Could you check a few things on this drawing? It's one solid part, dimensions in mm from its lowest x, y, z. A direction names the side the tool comes from. Round coordinates to 2 decimals unless told otherwise and drop trailing zeros. Order: outer loops, then holes, each group sorted by start corner. A loop starts at its lowest first (then second) coordinate and runs counter-clockwise, first axis right, second up.
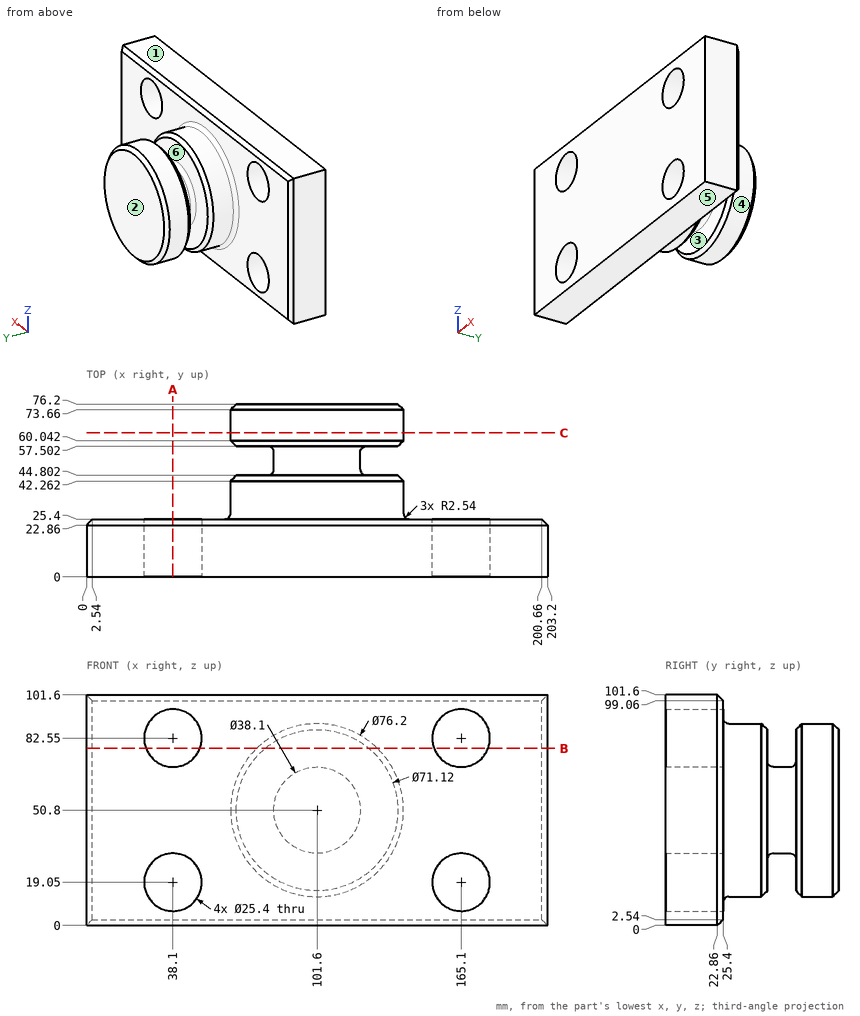
(1) I want a section at B-B, the plane z = 78. Give the number of separate pieces and of enclosed holes in the cut face, plus the area to 3 significant figures.
(2) I want a section at A-A, the plane x = 38.1. List the corners of the cut face in (y, z) for me, plus the area to 3 significant figures.
(3) I'm going to push flat-ended pins straight in: pin 1 Ø4 at (y, z) = (56, 67) entering from +X; pin 2 Ø2 at (x, z) = (132.5, 22.5) entering from -Y; pin 3 Ø1 at (y, z) = (50, 33.5) entering from -X; pin 4 Ø1.5 at (y, z) = (58, 21.5) entering from +X. Where does each tip first touch, or does it pass through?
(4) I want a section at C-C, the plane y = 63.5. List the corners of the cut face in (x, z) for me, plus the area to 3 significant figures.
(5) If we mould it in two halves opening along Y, with no side actions, what happens to the marked faces 1, 2 and 3? For each: pulls with the +Y half, pulls with the -Y half, needs draft (parallel to the pull), parting line crosses it, or undercut.
(6) On a 3-axis mill with a long thin cutter (end or side, diameter ignored), from which of +Z, -Z, +X, -X, +Y, -Y can I reach the whole of each face in a straight line? I mean the marked faces 4, 5 and 6. Say none if no direction works.
(7) Please list where these lines run through material, in increasing order: probe 1 along Z at (x, y) = (38.1, 7.5); probe 2 along X at (y, z) = (11, 82); probe 3 along X at (y, z) = (23.5, 83).
Ans:
1. separate pieces: 4
1. enclosed holes: 0
1. area: 5,960 mm2
2. outline: (0, 0) - (22.86, 0) - (25.4, 2.54) - (25.4, 6.35) - (0, 6.35) - close; (0, 31.75) - (25.4, 31.75) - (25.4, 69.85) - (0, 69.85) - close; (0, 95.25) - (25.4, 95.25) - (25.4, 99.06) - (22.86, 101.6) - (0, 101.6) - close
2. area: 1,280 mm2
3. pin 1: stops at x = 134.02
3. pin 2: stops at y = 0
3. pin 3: stops at x = 92.62
3. pin 4: stops at x = 124.22
4. outline: circle Ø76.2 at (101.6, 50.8)
4. area: 4,560 mm2
5. face 1: needs draft
5. face 2: pulls with the +Y half
5. face 3: undercut
6. face 4: +Y
6. face 5: -Z, +X, -X, +Y, -Y
6. face 6: none
7. probe 1: z = 0 to 6.35, 31.75 to 69.85, 95.25 to 101.6
7. probe 2: x = 0 to 25.41, 50.79 to 152.41, 177.79 to 203.2
7. probe 3: x = 0.64 to 25.41, 50.79 to 152.41, 177.79 to 202.56
